Autodesk Inventor part; units mm, degrees
ref_plane "YZ Plane" through (0, 0, 0) normal (1, 0, 0) x (0, 1, 0)
ref_plane "XZ Plane" through (0, 0, 0) normal (0, 1, 0) x (-1, 0, 0)
ref_plane "XY Plane" through (0, 0, 0) normal (0, 0, 1) x (1, 0, 0)
sketch "Sketch1" plane through (0, 0, 0) normal (0, 0, 1) x (1, 0, 0)
  ellipse E0 centre (-4.5001, 27.5565) end of major axis (-7.5001, 27.5565) minor radius 3
  line L0 (-2.0001, 9.3017) -> (-2.0001, 9.2846)
  line L1 (-2.0001, 45.8017) -> (-2.0001, 45.7846)
  line L2 (-1445.7599, 60) -> (10.4999, 60)
  line L3 (-19.4999, -29.9999) -> (-19.4999, 60)
  line L4 (10.4999, -29.9999) -> (10.4999, 60)
  line L5 (8.4999, -29.9999) -> (0, -29.9999)
  line L6 (10.4999, -29.9999) -> (-19.4999, -29.9999)
  line L7 (-19.4999, -29.9999) -> (-19.4999, 60)
  line L8 (-19.4999, 60) -> (10.4999, 60)
  line L9 (10.4999, 60) -> (10.4999, -29.9999)
  circle A0 centre (-4.5001, 27.5565) radius 4
  circle A1 centre (-4.5001, 45.8024) radius 2.5
  circle A2 centre (-4.5001, 9.3024) radius 2.5
  line L10 (-4.5, -29.9999) -> (-4.5, -14.9999) construction
  circle A3 centre (-4.5, -14.9999) radius 4
  point P0 (0, 0)
  dimension "d0" = 8
  dimension "d1" = 5
  dimension "d2" = 89.9999
  dimension "d3" = 15
  dimension "d4" = 8
extrude "Plate1" add sketch "Sketch1" along normal blind 2 contours L2 L4 L6 L5 L3
equation "\"BendRadius\" = Thickness"
equation "\"BendReliefWidth\" = Thickness"
equation "\"BendReliefDepth\" = 0.5 * Thickness"
equation "\"CornerReliefSize\" = 4 * Thickness"
equation "\"MinimumRemnant\" = 2 * Thickness"
equation "\"TransitionRadius\" = BendRadius"
equation "\"JacobiRadiusSize\" = BendRadius"
equation "\"GapSize\" = Thickness"
equation "\"d5\" = BendRadius"
properties part number "gabatarito-rolamento" material "Wood (Oak)"
Geometry: final body of the model. Coordinates: model frame, mm. Give positions to 0.01 mm unless a question says otherwise; leave off trailing zeros. Loops run counter-clockwise (first coordinate to the right, second up) from the corner with the lowest first, then second, coordinate; pieces in that order, holes last. Notation, with made-up numbers: (23.25, 68.25) - (44.25, 68.25) arc R13 ccw to (44.25, 73.25) - close; hole circle Ø5 at (83, 77). An arc over 180 degrees is marked (long way). Answer as CSV lines item,"result". Start each with the question number.
1. Section B-B, the plane z = 1.6. Give the number of separate pieces and of enclosed holes in the cut face, plus the area to 3 significant figures.
2. Ray query, L1, parallel to Y at x = -4.5, z = 1; L2, parallel to Y at x = -5.25, z = 0.6; L3, parallel to X at y = 45.5, z = 1.9. Return the intervals inside material, ascending.
3. Draft query along Y for faces 1 (the face through (-7, 9.2, 1)), 2 (the face through (-5.367, -11.095, 0.986)), 3 (the face through (-19.5, 14, 1)), 4 (the face through (-5, 60, 1)). Return one class per face: released by +Y, released by -Y, zero draft, split by the parting line, or undercut.
4. Section A-A, the plane x = -4.5. Return loops of the section in (y, z).
5. Section C-C, the plane y = 26. Return loops of the section in (x, z), plus the area to 3 significant figures.
6. Pin query (flat end, axial travel): P1, Ø5, axis at x = -4.5, y = 27.56, coming from the -Z side; P2, Ø8, axis at x = -4.5, y = 9.3, coming from the +Z side. Return the tip coordinate at first contact, or that it passes through.
Answers:
1,separate pieces,"1"
1,enclosed holes,"4"
1,area,"2,560 mm2"
2,L1,"y = -30 to -19, -11 to 6.8, 11.8 to 23.56, 31.56 to 43.3, 48.3 to 60"
2,L2,"y = -30 to -18.93, -11.07 to 6.92, 11.69 to 23.63, 31.49 to 43.42, 48.19 to 60"
2,L3,"x = -19.5 to -6.98, -2.02 to 10.5"
3,face 1,"undercut"
3,face 2,"undercut"
3,face 3,"zero draft"
3,face 4,"released by +Y"
4,outline,"(-30, 0) - (-19, 0) - (-19, 2) - (-30, 2) - close; (-11, 0) - (6.8, 0) - (6.8, 2) - (-11, 2) - close; (11.8, 0) - (23.56, 0) - (23.56, 2) - (11.8, 2) - close; (31.56, 0) - (43.3, 0) - (43.3, 2) - (31.56, 2) - close; (48.3, 0) - (60, 0) - (60, 2) - (48.3, 2) - close"
5,outline,"(-19.5, 0) - (-8.18, 0) - (-8.18, 2) - (-19.5, 2) - close; (-0.82, 0) - (10.5, 0) - (10.5, 2) - (-0.82, 2) - close"
5,area,"45.3 mm2"
6,P1,"passes through"
6,P2,"stops at z = 2"
